```python
from build123d import *

# Parameters (mm, degrees)
F1_DEPTH = 6.35
F4_W     = 127
F4_H     = 147.3902405336
F4_W_2   = 114.3
F4_H_2   = 131.6580059171
F5_DEPTH = 6.35
F6_W     = 146.5334397942
F6_H     = 127
F6_W_2   = 133.8334397942
F6_H_2   = 114.3
F7_DEPTH = 6.35
F8_R     = 38.1
F9_DEPTH = 20.32


with BuildPart() as f1:
    # F0 (on Front) → F1 (new body)
    with BuildSketch(Plane.XZ):
        with BuildLine():
            Line((146.5334397942, -6.35), (146.5334397942, 69.85))
            Line((146.5334397942, 69.85), (92.6519030678, 123.7315367264))
            Line((92.6519030678, 123.7315367264), (-10.9628858813, 20.1167477774))
            ThreePointArc((-10.9628858813, 20.1167477774), (-12.7007443513, 16.8654432616), (-12.3393928522, 13.1965799213))
            Line((-12.3393928522, 13.1965799213), (-5.8666350314, -2.4300397955))
            ThreePointArc((-5.8666350314, -2.4300397955), (-3.5278709797, -5.2798320381), (0, -6.35))
            Line((0, -6.35), (146.5334397942, -6.35))
        make_face()
        Polygon((140.1834397942, 0), (0, 0), (-2.0213590126, 4.8799923427), (140.1834397942, 63.783148643), align=None, mode=Mode.SUBTRACT)
        Polygon((-4.4513988081, 10.7466273741), (-6.4727578208, 15.6266197168), (92.6519030678, 114.7512806053), (137.7533999987, 69.6497836744), align=None, mode=Mode.SUBTRACT)
    extrude(amount=F1_DEPTH)


with BuildPart() as f3_1:
    # F3: instance of F1
    add(f1.part.mirror(Plane.XZ.offset(-57.15)))


with BuildPart() as f1_1:
    add(f1.part)

    add(f3_1.part)  # F5 merges F3_1
    # F4 (on face) → F5 (join)
    with BuildSketch(Plane(origin=(-15.5398168293, 0, 15.5398168293), x_dir=(0, -1, 0), z_dir=(-0.7071067812, 0, 0.7071067812))):
        with Locations((-57.15, 79.3110773481)):
            Rectangle(F4_W, F4_H)
        with Locations((-57.15, 77.7949600399)):
            Rectangle(F4_W_2, F4_H_2, mode=Mode.SUBTRACT)
        Polygon((6.35, 153.0061976149), (-114.3, 153.0061976149), (-114.3, 143.6239629984), (0, 143.6239629984), (0, 11.9659570813), (-114.3, 11.9659570813), (-114.3, 6.4727578208), (-120.65, 6.4727578208), (-120.65, 5.6159570813), (6.35, 5.6159570813), align=None)
    extrude(amount=-F5_DEPTH)

    # F6 (on face) → F7 (join)
    with BuildSketch(Plane(origin=(0, 0, -6.35), x_dir=(1, 0, 0), z_dir=(0, 0, -1))):
        with Locations((73.2667198971, -57.15)):
            Rectangle(F6_W, F6_H)
        with Locations((73.2667198971, -57.15)):
            Rectangle(F6_W_2, F6_H_2, mode=Mode.SUBTRACT)
    extrude(amount=-F7_DEPTH)

    # F8 (on face) → F9 (join)
    with BuildSketch(Plane.XZ.offset(-114.3)):
        with Locations((39.2216469467, 25.4)):
            Circle(F8_R)
    extrude(amount=F9_DEPTH)

    # F10: F1 across plane


with BuildPart() as f1_2:
    add(f1_1.part)
    add(f1_1.part.mirror(Plane.XZ.offset(-57.15)))


solid = f1_2.part
```
Can you work these out from the model? Positions are in its coordinate system, mm. A direction names the side the tool comes from. Give positions to 0.01 mm unless a question says otherwise; leave off trailing zeros. Order: outer loops, then holes, each group sorted by start corner. A loop starts at its lowest first (then second) coordinate and runs counter-clockwise, first axis right, second up. Notation, with made-up numbers: M -21,-2 L 37,-2 A18 cw 37,30 Z; hole C 64.5,1.25 d3. An arc over 180 degrees is marked long. Write item = value, one per line. Start each with the question number.
Q1. Will these pins go through, and if not, where does the flat tip stop? pin 1 Ø7 at (y, z) = (81.5, -5) entering from -X; pin 2 Ø5 at (x, y) = (142, 60.5) entering from +Z; pin 3 Ø1.5 at (y, z) = (23, 15) entering from -X.
Q2. I need wall thicknesses on probe 1 along Y at (x, z) = (43, 25.5); probe 2 along Z at (x, y) = (113.5, 115.5). Which ranges of each line are inside material? Lowest first, please. Write a range as [from, to].
Q3. For faces 4 (the flat face through (37, 0, 39)), 5 (the flat face through (-4.865, 57.95, 21.787)), 6 (the flat face through (49, 114.3, 15)), 7 (the cylindrical face through (56.802, 10.018, -8.401)), 8 (the flat face through (-5.448, 117.431, 13.152)), which set-ups out of +Z, -Z, +X, -X, +Y, -Y let a thin tool reach every point of the face, with its end or its side?
Q4. Suppose I cut it at A-A (y = 63). Write out the boundary of the cut face in (x, z).
Q5. We'd pull the mould along Z, two halves only. Please class faces 1 (the flat face through (39, 93.98, 26)), 2 (the flat face through (87.105, 57.446, 118.185)), 3 (the flat face through (68.09, 117.43, 33.92)): pulls with the +Z half, pulls with the -Z half, needs draft (parallel to the pull), parting line crosses it, or undercut.
Q6. Suppose I cut it at B-B (x = 65.5). Count the separate pieces of the cut face and the enclosed holes in it, plus the area to 3 significant figures.
Q7. Suppose I cut it at C-C (z = 98.5). Write out the boundary of the cut face in (x, y), plus the area to 3 significant figures.
Check result:
q1.pin_1 = 0
q1.pin_2 = 0
q1.pin_3 = -7.81
q2.probe_1 = [-6.35, 20.32], [93.98, 120.65]
q2.probe_2 = [-6.35, 0], [52.73, 59.6], [93.9, 102.88]
q3.face_4 = -Y
q3.face_5 = +Z
q3.face_6 = +Y
q3.face_7 = none
q3.face_8 = +Y, -Y
q4.outline = M -11.57,19.51 L -7.08,15.02 L -2.59,19.51 L -7.08,24 Z; M 0,-6.35 L 6.35,-6.35 L 6.35,0 L 0,0 Z; M 86.02,117.1 L 90.51,112.61 L 97.14,119.24 L 92.65,123.73 Z; M 140.18,-6.35 L 146.53,-6.35 L 146.53,0 L 140.18,0 Z
q5.face_1 = needs draft
q5.face_2 = pulls with the +Z half
q5.face_3 = undercut
q6.separate_pieces = 4
q6.enclosed_holes = 0
q6.area = 2,520 mm2
q7.outline = M 67.42,-6.35 L 76.4,-6.35 L 76.4,0 L 67.42,0 Z; M 67.42,114.3 L 76.4,114.3 L 76.4,120.65 L 67.42,120.65 Z; M 108.9,-6.35 L 117.88,-6.35 L 117.88,0 L 108.9,0 Z; M 108.9,114.3 L 117.88,114.3 L 117.88,120.65 L 108.9,120.65 Z
q7.area = 228 mm2
